```python
from build123d import *

# Parameters (mm, degrees)
SKETCH1_R            = 18
BOSS_EXTRUDE1_DEPTH  = 10
SKETCH2_R            = 2
BOSS_EXTRUDE11_DEPTH = 1
SKETCH3_R            = 2
CUT_EXTRUDE1_DEPTH   = 2


with BuildPart() as part:
    # Sketch1 → Boss-Extrude1 (new body)
    with BuildSketch(Plane(origin=(0, 0, 0), x_dir=(1, 0, 0), z_dir=(0, 1, 0))):
        with Locations(Location((0, 0, 0), (0, 0, 270))):
            Circle(SKETCH1_R)
    extrude(amount=BOSS_EXTRUDE1_DEPTH)

    # Sketch2 → Boss-Extrude11 (add)
    with BuildSketch(Plane.XZ):
        with BuildLine():
            ThreePointArc((-12.727922061, -12.727922061), (-16.629831585, -6.888301783), (-18, 0))
            ThreePointArc((-18, 0), (-16.629831585, 6.888301783), (-12.727922061, 12.727922061))
            add(Edge.make_bspline(
                [(-12.727922061, 12.727922061), (-17.413514116, 10.578941286), (-22.725992236, 6.653009013), (-24.419739959, 2.952843449), (-24.810237614, 1.3644098)],
                knots=[0, 0, 0, 0, 0.294966877, 0.815844303, 0.815844303, 0.815844303, 0.815844303], degree=3))
            add(Edge.make_bspline(
                [(-24.810237614, 1.3644098), (-24.948297671, 0.80282066), (-25, 0.337972177), (-25, 0)],
                knots=[0.815844303, 0.815844303, 0.815844303, 0.815844303, 1, 1, 1, 1], degree=3))
            add(Edge.make_bspline(
                [(-24.810237614, -1.3644098), (-24.948297671, -0.80282066), (-25, -0.337972177), (-25, 0)],
                knots=[0.815844303, 0.815844303, 0.815844303, 0.815844303, 1, 1, 1, 1], degree=3))
            add(Edge.make_bspline(
                [(-12.727922061, -12.727922061), (-17.413514116, -10.578941286), (-22.725992236, -6.653009013), (-24.419739959, -2.952843449), (-24.810237614, -1.3644098)],
                knots=[0, 0, 0, 0, 0.294966877, 0.815844303, 0.815844303, 0.815844303, 0.815844303], degree=3))
        make_face()
        with Locations((-20, 0)):
            Circle(SKETCH2_R, mode=Mode.SUBTRACT)
        with Locations((-20, 0)):
            Circle(SKETCH2_R)
        with BuildLine():
            ThreePointArc((12.727922061, 12.727922061), (16.629831585, 6.888301783), (18, 2e-09))
            ThreePointArc((18, 2e-09), (16.629831586, -6.888301782), (12.727922061, -12.727922061))
            add(Edge.make_bspline(
                [(12.727922061, -12.727922061), (17.413514116, -10.578941286), (23.925146422, -5.766831599), (25, -1.293913703), (25, 0)],
                knots=[0, 0, 0, 0, 0.294966877, 1, 1, 1, 1], degree=3))
            add(Edge.make_bspline(
                [(12.727922061, 12.727922061), (17.413514116, 10.578941286), (23.925146422, 5.766831599), (25, 1.293913703), (25, 0)],
                knots=[0, 0, 0, 0, 0.294966877, 1, 1, 1, 1], degree=3))
        make_face()
        with BuildLine():
            ThreePointArc((18, 2e-09), (20.000000001, 2), (22, 0))
            ThreePointArc((22, 0), (19.999999999, -2), (18, 2e-09))
        make_face(mode=Mode.SUBTRACT)
        with BuildLine():
            ThreePointArc((18, 2e-09), (19.999999999, -2), (22, 0))
            ThreePointArc((22, 0), (20.000000001, 2), (18, 2e-09))
        make_face()
    extrude(amount=-BOSS_EXTRUDE11_DEPTH)

    # Sketch3 → Cut-Extrude1 (cut)
    with BuildSketch(Plane.XZ):
        with Locations(Location((-20, 0, 0), (0, 0, 270))):
            Circle(SKETCH3_R)
        with Locations(Location((20, 0, 0), (0, 0, 270))):
            Circle(SKETCH3_R)
    extrude(amount=-CUT_EXTRUDE1_DEPTH, mode=Mode.SUBTRACT)

    # Sketch4 → Revolve1 (revolve)
    with BuildSketch(Plane(origin=(0, 10, 0), x_dir=(1, 0, 0), z_dir=(0, 1, 0))):
        with BuildLine():
            Line((0, 10), (0, -10))
            ThreePointArc((0, -10), (10, 0), (0, 10))
        make_face()
    revolve(axis=Axis((0, 10, -19.956600841), (0, 0, 1)))


solid = part.part
```
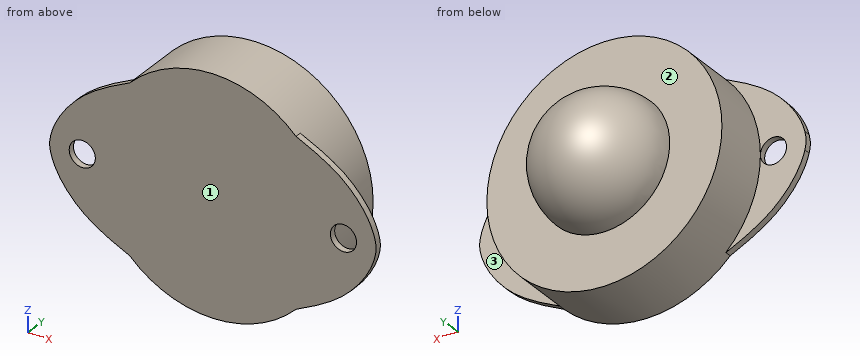
Here's how the part is built. I have some questions about the finished solid (model axes, mm). Face numbers are marked on the shaded views. A direction names the side the tool comes from. Coordinates: 2 decimals unless noted, no trailing zeros. Order: outer loops, then holes, each group sorted by start corner. A loop starts at its lowest first (then second) coordinate and runs counter-clockwise, first axis right, second up. Notation, with made-up numbers: M 47.25,-8 L 94.25,-8 A7 cw 94.25,1 Z; hole C 49,-31.75 d4. An arc over 180 degrees is marked long. Answer as a JSON object with one key per item and string values. Group by question number.
(1) Which directions (+Z, -Z, +X, -X, +Y, -Y) give clear straight access to the entire face, cutting with the end or side of a thin tool? Please do the marked faces 1, 2 and 3.
(2) For pin 1 (3.5 mm diameter, centred on x = 20, z = 0, fed in from -Y); pin 2 (10 mm diameter, centred on x = -1, z = -11, fed in from +Y); pin 3 (3 mm diameter, centred on y = 4, z = 1.5, fed in from -X); pin 4 (8 mm diameter, centred on x = 14, y = 11.5, fed in from -Z), each with a flat end and sliding along its axis, tell me the tip position at first contact or that it passes through.
(3) Suppose I cut it at A-A, the plane x = 0. Please give me the cut outline in (y, z).
(4) Suppose I cut it at C-C, the plane z = -14. Please give me the cut outline in (x, y), then the cut area to 3 significant figures.
(5) Suppose I cut it at D-D, the plane y = 13. Please give me the cut outline in (x, z).
(6) Suppose I cut it at B-B, the plane y = 6. Please give me the cut outline in (x, z), then the cut area to 3 significant figures.
(7) I need wall thicknesses on probe 1 along X at (y, z) = (0.55, 0); probe 2 along Y at (x, z) = (18, 2.5); probe 3 along Y at (x, z) = (-8, 15). Which ranges of each line are inside material? Lowest first, please.
Values found:
{
 "1": {"face 1": "+Z, -Z, +X, -X, -Y", "face 2": "+Y", "face 3": "+X, +Y"},
 "2": {"pin 1": "passes through", "pin 2": "stops at y = 17.97", "pin 3": "stops at x = -18", "pin 4": "stops at z = -14.77"},
 "3": {"outline": "M 0,-18 L 10,-18 L 10,-10 A10 ccw 10,10 L 10,18 L 0,18 Z"},
 "4": {"outline": "M -11.31,0 L 11.31,0 L 11.31,10 L -11.31,10 Z", "area": "226 mm^2"},
 "5": {"outline": "C 0,0 d19.08"},
 "6": {"outline": "C 0,0 d36", "area": "1,020 mm^2"},
 "7": {"probe 1": "x = -25 to -22, -18 to 18, 22 to 25", "probe 2": "y = 0 to 1", "probe 3": "y = 0 to 10"}
}
